Read the model definition and answer for the solid it produces. Units are mm, in the model's axes. A direction names the side the tool comes from. Round coordinates to 2 decimals unless told otherwise and drop trailing zeros. Order: outer loops, then holes, each group sorted by start corner. A loop starts at its lowest first (then second) coordinate and runs counter-clockwise, first axis right, second up. Notation, with made-up numbers: (-10.75, 18.5) -> (6.25, 18.5) arc R9 cw to (6.25, 32.5) -> close; hole circle Ø10 at (19, 4). An arc over 180 degrees is marked (long way). Answer as a JSON object with one key per item and string values. Group by question number.
Item 1: Consider probe 1 along Y at (x, z) = (-4.5, -6.75); probe 2 along Z at (x, y) = (-6.25, -1.5); probe 3 along Z at (x, y) = (5, 2.5). Determine where each line is inside the solid, lowest interval first. Write a range as from..to.
Item 2: For faces 1 (the flat face through (0, 11, 0)), 2 (the cylindrical face through (0, 8, -1)), determine the directions among +Z, -Z, +X, -X, +Y, -Y from which every point of the face is accessible in a straight line to the end or side of a thin tool.
Item 3: Section C-C, the plane y = 3 is taken. Write down the section's boundary in (x, z), plus the area to 3 significant figures.
Item 4: Section A-A, the plane x = 0 is taken. Write down the section's boundary in (y, z).
Item 5: Section B-B, the plane z = 0 is taken. Write down the section's boundary in (x, y).
Item 6: Given P1, Ø3, axis at x = 4, z = 8.5, coming from the +Y side; P2, Ø5, axis at y = -3.5, z = 7, coming from the -X side, each flat-ended and moving along its own axis, determine where each tip first touches the part or whether it passes through.
Item 7: Section D-D, the plane x = -8.5 is taken. Write down the section's boundary in (y, z).
from build123d import *

# Parameters (mm, degrees)
F0_R     = 13
F0_R_2   = 11.5
F1_DEPTH = 6
F2_DEPTH = 6
F3_R     = 1
F4_DEPTH = 5


with BuildPart() as f1:
    # F0 (on Front) → F1 (new body, symmetric)
    with BuildSketch(Plane.XZ):
        Circle(F0_R)
        Circle(F0_R_2, mode=Mode.SUBTRACT)
    extrude(amount=F1_DEPTH, both=True)

    # F0 (on Front) → F2 (join, symmetric)
    with BuildSketch(Plane.XZ):
        Circle(F0_R_2)
    extrude(amount=F2_DEPTH, both=True)

    # F3 (on face) → F4 (join)
    with BuildSketch(Plane(origin=(0, 6, 0), x_dir=(-1, 0, 0), z_dir=(0, 1, 0))):
        Circle(F3_R)
    extrude(amount=F4_DEPTH)


solid = f1.part
Values found:
{
 "1": {"probe 1": "-6..6", "probe 2": "-11.4..11.4", "probe 3": "-12..12"},
 "2": {"face 1": "+Z, -Z, +X, -X, +Y", "face 2": "+Y"},
 "3": {"outline": "circle Ø26 at (0, 0)", "area": "531 mm2"},
 "4": {"outline": "(-6, -13) -> (6, -13) -> (6, -1) -> (11, -1) -> (11, 1) -> (6, 1) -> (6, 13) -> (-6, 13) -> close"},
 "5": {"outline": "(-13, -6) -> (13, -6) -> (13, 6) -> (1, 6) -> (1, 11) -> (-1, 11) -> (-1, 6) -> (-13, 6) -> close"},
 "6": {"P1": "y = 6", "P2": "x = -12.2"},
 "7": {"outline": "(-6, -9.84) -> (6, -9.84) -> (6, 9.84) -> (-6, 9.84) -> close"}
}
